from build123d import *

# Parameters (mm, degrees)
EXTRUDE_2_DEPTH     = 14
FILLET_1_RADIUS     = 7
FILLET_1_LENGTH     = 6.553419282
FILLET_2_RADIUS     = 7
FILLET_2_LENGTH     = 6.553419282
CUT_EXTRUDE_1_REACH = 142.851
SKETCH_2_R          = 2.15
EXTRUDE_3_DEPTH     = 14
FILLET_3_RADIUS     = 7
FILLET_3_LENGTH     = 6
FILLET_4_RADIUS     = 7
FILLET_4_LENGTH     = 6
EXTRUDE_5_REACH     = 144.825
SKETCH_8_R          = 2.5
SKETCH_8_W          = 40.683862831
SKETCH_8_H          = 14
EXTRUDE_6_REACH     = 144.34
SKETCH_11_R         = 2.5
SKETCH_12_W         = 25
SKETCH_12_H         = 14
EXTRUDE_7_DEPTH     = 12
SKETCH_13_R         = 5
CUT_EXTRUDE_2_DEPTH = 12
FILLET_5_R          = 5


with BuildPart() as part:
    # Sketch 1 → Extrude 2 (new body)
    with BuildSketch(Plane(origin=(0, 0, 0), x_dir=(1, 0, 0), z_dir=(0, 1, 0))):
        with BuildLine():
            Line((5, 0), (5, 62.718048915))
            ThreePointArc((5, 62.718048915), (4.918829182, 63.989594298), (4.676634468, 65.240497206))
            Line((4.676634468, 65.240497206), (2.323365532, 74.268124597))
            ThreePointArc((2.323365532, 74.268124597), (2.081170818, 75.519027505), (2, 76.790572889))
            Line((2, 76.790572889), (2, 140))
            Line((2, 140), (-4.553419282, 140))
            Line((-4.553419282, 140), (-4.553419282, 76.790572889))
            ThreePointArc((-4.553419282, 76.790572889), (-4.472248464, 75.519027505), (-4.23005375, 74.268124597))
            Line((-4.23005375, 74.268124597), (-1.876784815, 65.240497206))
            ThreePointArc((-1.876784815, 65.240497206), (-1.6345901, 63.989594298), (-1.553419282, 62.718048915))
            Line((-1.553419282, 62.718048915), (-1.553419282, 0))
            Line((-1.553419282, 0), (5, 0))
        make_face()
    extrude(amount=EXTRUDE_2_DEPTH)

    # Fillet 1: full round fillet: the end face becomes a half cylinder, R = half its width
    fillet_1_face = Plane((1.723290359, 7, 0), x_dir=(1, 0, 0), z_dir=(0, 0, 1))  # on the end face: x along it, z out of the body
    fillet_1_slab = fillet_1_face.offset(-FILLET_1_RADIUS / 2) * Box(FILLET_1_LENGTH, 2 * FILLET_1_RADIUS, FILLET_1_RADIUS, mode=Mode.PRIVATE)  # the body's end, R deep
    fillet_1_round = Plane((1.723290359, 7, -7), x_dir=(0, 0, 1), z_dir=(1, 0, 0)) * Cylinder(FILLET_1_RADIUS, FILLET_1_LENGTH, mode=Mode.PRIVATE)  # its axis R under the face
    add(fillet_1_slab - fillet_1_round, mode=Mode.SUBTRACT)

    # Fillet 2: full round fillet: the end face becomes a half cylinder, R = half its width
    fillet_2_face = Plane((-1.276709641, 7, -140), x_dir=(-1, 0, 0), z_dir=(0, 0, -1))  # on the end face: x along it, z out of the body
    fillet_2_slab = fillet_2_face.offset(-FILLET_2_RADIUS / 2) * Box(FILLET_2_LENGTH, 2 * FILLET_2_RADIUS, FILLET_2_RADIUS, mode=Mode.PRIVATE)  # the body's end, R deep
    fillet_2_round = Plane((-1.276709641, 7, -133), x_dir=(0, 0, -1), z_dir=(-1, 0, 0)) * Cylinder(FILLET_2_RADIUS, FILLET_2_LENGTH, mode=Mode.PRIVATE)  # its axis R under the face
    add(fillet_2_slab - fillet_2_round, mode=Mode.SUBTRACT)

    # Sketch 2 → Cut-Extrude 1 (cut, up to next)
    with BuildSketch(Plane(origin=(2, 0, 0), x_dir=(0, 0, -1), z_dir=(1, 0, 0)), mode=Mode.PRIVATE) as cut_extrude_1_sk1:
        with Locations((133, 7)):
            Circle(SKETCH_2_R)
    cut_extrude_1_tool1 = extrude(cut_extrude_1_sk1.sketch, amount=-CUT_EXTRUDE_1_REACH, mode=Mode.PRIVATE) & part.part
    add(cut_extrude_1_tool1.solids().sort_by_distance((2, 7, -133))[0], mode=Mode.SUBTRACT)

    # Sketch 8 → Extrude 5 (add, up to next)
    with BuildSketch(Plane(origin=(-19.553419282, 0, 0), x_dir=(0, 0, -1), z_dir=(1, 0, 0)), mode=Mode.PRIVATE) as extrude_5_sk1:
        with Locations(Location((7, 7, 0), (0, 0, 180))):
            Circle(SKETCH_8_R)
    extrude_5_tool1 = extrude(extrude_5_sk1.sketch, amount=EXTRUDE_5_REACH, mode=Mode.PRIVATE) - part.part
    # Sketch 8 → Extrude 5 (add, up to next)
    with BuildSketch(Plane(origin=(-19.553419282, 0, 0), x_dir=(0, 0, -1), z_dir=(1, 0, 0)), mode=Mode.PRIVATE) as extrude_5_sk2:
        with Locations((42.341931415, 7)):
            Rectangle(SKETCH_8_W, SKETCH_8_H)
    extrude_5_tool2 = extrude(extrude_5_sk2.sketch, amount=EXTRUDE_5_REACH, mode=Mode.PRIVATE) - part.part


with BuildPart() as body_2:
    # Sketch 4 → Extrude 3 (new body)
    with BuildSketch(Plane(origin=(0, 0, 0), x_dir=(1, 0, 0), z_dir=(0, 1, 0))):
        with BuildLine():
            Line((-19.553419282, 0), (-25.553419282, 0))
            Line((-25.553419282, 0), (-25.553419282, 62.683862831))
            ThreePointArc((-25.553419282, 62.683862831), (-25.467917646, 63.988746812), (-25.212874842, 65.271316849))
            Line((-25.212874842, 65.271316849), (-22.893963723, 73.928250938))
            ThreePointArc((-22.893963723, 73.928250938), (-22.638920919, 75.210820976), (-22.553419282, 76.515704957))
            Line((-22.553419282, 76.515704957), (-22.553419282, 140))
            Line((-22.553419282, 140), (-16.553419282, 140))
            Line((-16.553419282, 140), (-16.553419282, 76.515704957))
            ThreePointArc((-16.553419282, 76.515704957), (-16.638920919, 75.210820976), (-16.893963723, 73.928250938))
            Line((-16.893963723, 73.928250938), (-19.212874842, 65.271316849))
            ThreePointArc((-19.212874842, 65.271316849), (-19.467917646, 63.988746812), (-19.553419282, 62.683862831))
            Line((-19.553419282, 62.683862831), (-19.553419282, 0))
        make_face()
    extrude(amount=EXTRUDE_3_DEPTH)

    # Fillet 3: full round fillet: the end face becomes a half cylinder, R = half its width
    fillet_3_face = Plane((-19.553419282, 7, -140), x_dir=(-1, 0, 0), z_dir=(0, 0, -1))  # on the end face: x along it, z out of the body
    fillet_3_slab = fillet_3_face.offset(-FILLET_3_RADIUS / 2) * Box(FILLET_3_LENGTH, 2 * FILLET_3_RADIUS, FILLET_3_RADIUS, mode=Mode.PRIVATE)  # the body's end, R deep
    fillet_3_round = Plane((-19.553419282, 7, -133), x_dir=(0, 0, -1), z_dir=(-1, 0, 0)) * Cylinder(FILLET_3_RADIUS, FILLET_3_LENGTH, mode=Mode.PRIVATE)  # its axis R under the face
    add(fillet_3_slab - fillet_3_round, mode=Mode.SUBTRACT)

    # Fillet 4: full round fillet: the end face becomes a half cylinder, R = half its width
    fillet_4_face = Plane((-22.553419282, 7, 0), x_dir=(1, 0, 0), z_dir=(0, 0, 1))  # on the end face: x along it, z out of the body
    fillet_4_slab = fillet_4_face.offset(-FILLET_4_RADIUS / 2) * Box(FILLET_4_LENGTH, 2 * FILLET_4_RADIUS, FILLET_4_RADIUS, mode=Mode.PRIVATE)  # the body's end, R deep
    fillet_4_round = Plane((-22.553419282, 7, -7), x_dir=(0, 0, 1), z_dir=(1, 0, 0)) * Cylinder(FILLET_4_RADIUS, FILLET_4_LENGTH, mode=Mode.PRIVATE)  # its axis R under the face
    add(fillet_4_slab - fillet_4_round, mode=Mode.SUBTRACT)


with BuildPart() as part_1:
    add(part.part)

    add(body_2.part)  # Extrude 5 merges body 2
    add(extrude_5_tool1.solids().sort_by_distance((-19.553419, 7, -7))[0])
    add(extrude_5_tool2.solids().sort_by_distance((-19.553419, 7, -42.341931))[0])

    # Sketch 11 → Extrude 6 (add, up to next)
    with BuildSketch(Plane(origin=(-16.553419282, 0, 0), x_dir=(0, 0, -1), z_dir=(1, 0, 0)), mode=Mode.PRIVATE) as extrude_6_sk1:
        with Locations(Location((103.7, 7, 0), (0, 0, 180))):
            Circle(SKETCH_11_R)
    extrude_6_tool1 = extrude(extrude_6_sk1.sketch, amount=EXTRUDE_6_REACH, mode=Mode.PRIVATE) - part_1.part
    add(extrude_6_tool1.solids().sort_by_distance((-16.553419, 7, -103.7))[0])

    # Sketch 12 → Extrude 7 (add)
    with BuildSketch(Plane(origin=(-16.553419282, 0, 0), x_dir=(0, 0, -1), z_dir=(1, 0, 0))):
        with Locations((142.898160933, 7)):
            Rectangle(SKETCH_12_W, SKETCH_12_H)
    extrude(amount=EXTRUDE_7_DEPTH)

    # Sketch 13 → Cut-Extrude 2 (cut)
    with BuildSketch(Plane.ZY.offset(16.553419282)):
        with Locations((-147.398160933, 7)):
            Circle(SKETCH_13_R)
    extrude(amount=-CUT_EXTRUDE_2_DEPTH, mode=Mode.SUBTRACT)

    # Fillet 5
    fillet_5_edges = [part_1.edges().sort_by_distance(p)[0] for p in [
        (-10.553419282, 0, -155.398160933),
        (-10.553419282, 14, -155.398160933),
    ]]
    fillet(fillet_5_edges, radius=FILLET_5_R)


solid = part_1.part
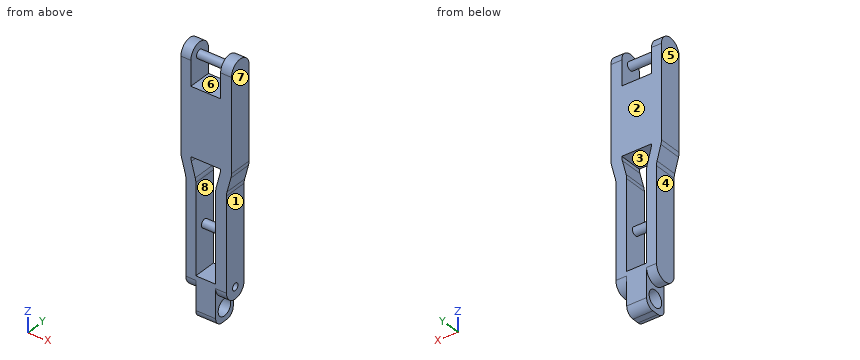
Can you work these out from the model? Positions are in its coordinate system, mm. Face numbers are marked on the shaded views. A direction names the side the tool comes from. Coordinates: 2 decimals unless noted, no trailing zeros. Loops run counter-clockwise (first coordinate to the right, second up) from the corner with the lowest first, then second, coordinate; pieces in that order, holes last. Notation, with made-up numbers: M 26.5,42.25 L 84.5,42.25 A23 cw 84.5,74.25 Z; hole C 84,27 d2. An arc over 180 degrees is marked long. Return JSON: item names as keys, results as strings. Group by question number.
Item 1: Imagine slicing it at C-C (y = 7). Give the number of separate pieces and of enclosed holes in the cut face, and give its area (3 significant figures).
Item 2: If I drill on L1, parallel to Y at x = 0, z = -133; L2, parallel to X at y = 10, z = -111; L3, parallel to X at y = 2.5, z = -63, over which ranges is the centre line in solid material (lowest first)? Write a range as from..to.
Item 3: Thinking about a two-plate mould opening in Z: for the marked faces 6, 7 and 8, which applies, released by +Z, released by -Z, zero draft, split by the parting line, or undercut?
Item 4: Imagine slicing it at A-A (x = -12). Please give me the cut outline in (y, z).
Item 5: I'm going to push flat-ended pins straight in: pin 1 Ø4 at (y, z) = (3.5, -100) entering from +X; pin 2 Ø4 at (y, z) = (4, -111.5) entering from -X; pin 3 Ø7 at (y, z) = (7.5, -148) entering from -X; pin 4 Ø7 at (x, y) = (-8.5, 9) entering from +Z. Where does each tip first touch, or does it pass through?
Item 6: On a 3-axis mill with a long thin cutter (end or side, diameter ignored), from which of +Z, -Z, +X, -X, +Y, -Y can I reach the whole of each face in a straight line? I mean the marked faces 1, 2, 3, 4 and 5. Say none if no direction works.
Item 7: Imagine slicing it at D-D (z = -136.5). Please give me the cut outline in (x, y), and give its area (3 significant figures).
Item 8: Imagine slicing it at B-B (z = -97). Please give me the cut outline in (x, y).
Verdict:
{
 "1": {"separate pieces": "2", "enclosed holes": "3", "area": "2,790 mm^2"},
 "2": {"L1": "y = 0..4.85, 9.15..14", "L2": "x = -22.55..-16.55, -4.55..2", "L3": "x = -25.55..-19.55, -1.56..5"},
 "3": {"face 6": "undercut", "face 7": "zero draft", "face 8": "undercut"},
 "4": {"outline": "M 0,-150.4 A5 ccw 5,-155.4 L 9,-155.4 A5 ccw 14,-150.4 L 14,-130.4 L 0,-130.4 Z; M 0,-62.68 L 14,-62.68 L 14,-22 L 0,-22 Z; C 7,-103.7 d5; C 7,-7 d5; hole C 7,-147.4 d10"},
 "5": {"pin 1": "stops at x = 2", "pin 2": "stops at x = -22.55", "pin 3": "passes through", "pin 4": "stops at z = -4.5"},
 "6": {"face 1": "-Z, +X, +Y, -Y", "face 2": "+Z, -Z, +X, -X, +Y", "face 3": "+Y, -Y", "face 4": "-Z, -X, +Y, -Y", "face 5": "+Z, -Z, -X, +Y, -Y"},
 "7": {"outline": "M -22.55,0.94 L -16.55,0.94 L -16.55,0 L -4.55,0 L -4.55,0.94 L 2,0.94 L 2,13.06 L -4.55,13.06 L -4.55,14 L -16.55,14 L -16.55,13.06 L -22.55,13.06 Z", "area": "320 mm^2"},
 "8": {"outline": "M -22.55,0 L -16.55,0 L -16.55,14 L -22.55,14 Z; M -4.55,0 L 2,0 L 2,14 L -4.55,14 Z"}
}
